from build123d import *

# Parameters (mm, degrees)
SKETCH1_W                 = 134.5
SKETCH1_H                 = 85
BOSS_EXTRUDE1_DEPTH       = 3
SKETCH2_W                 = 140.5
SKETCH2_H                 = 91
SKETCH2_W_2               = 134.5
SKETCH2_H_2               = 85
BOSS_EXTRUDE2_DEPTH       = 70
BOSS_EXTRUDE3_START       = 5
SKETCH3_W                 = 100
SKETCH3_H                 = 80
BOSS_EXTRUDE3_DEPTH       = 5
SKETCH5_W                 = 3
SKETCH5_H                 = 66
BOSS_EXTRUDE5_DEPTH       = 30
SKETCH6_R                 = 3
SKETCH6_R_2               = 1
BOSS_EXTRUDE6_DEPTH       = 10
SKETCH7_W                 = 100
SKETCH7_H                 = 80
CUT_EXTRUDE2_DEPTH        = 10
SKETCH6_2_R               = 3
SKETCH6_2_R_2             = 1
BOSS_EXTRUDE7_DEPTH       = 8
MIRROR4_COPY_1_SKETCH_R   = 3
MIRROR4_COPY_1_SKETCH_R_2 = 1
MIRROR4_COPY_1_DEPTH      = 8
SKETCH9_R                 = 26.15
SKETCH9_W                 = 29.3
SKETCH9_H                 = 26.2
SKETCH9_R_2               = 1
SKETCH9_R_3               = 3.4
SKETCH9_R_4               = 7.9
CUT_EXTRUDE3_DEPTH        = 3
SKETCH10_R                = 2.95
SKETCH10_R_2              = 5.9
CUT_EXTRUDE4_DEPTH        = 3
BOSS_EXTRUDE8_DEPTH       = 7
FILLET1_R                 = 4
CUT_EXTRUDE6_DEPTH        = 5


with BuildPart() as part:
    # Sketch1 → Boss-Extrude1 (new body)
    with BuildSketch(Plane(origin=(0, 0, 0), x_dir=(1, 0, 0), z_dir=(0, 1, 0))):
        with Locations((-12.25, 0)):
            Rectangle(SKETCH1_W, SKETCH1_H)
    extrude(amount=BOSS_EXTRUDE1_DEPTH)

    # Sketch2 → Boss-Extrude2 (add)
    with BuildSketch(Plane(origin=(0, 0, 0), x_dir=(1, 0, 0), z_dir=(0, 1, 0))):
        with Locations((-12.25, 0)):
            Rectangle(SKETCH2_W, SKETCH2_H)
        with Locations((-12.25, 0)):
            Rectangle(SKETCH2_W_2, SKETCH2_H_2, mode=Mode.SUBTRACT)
    extrude(amount=BOSS_EXTRUDE2_DEPTH)

    # Sketch5 → Boss-Extrude5 (add)
    with BuildSketch(Plane(origin=(0, 3, 0), x_dir=(1, 0, 0), z_dir=(0, 1, 0))):
        Polygon((-58, -26.5), (-58, -23.5), (-61, -23.5), (-79.5, -23.5), (-79.5, -26.5), align=None)
        with Locations((-59.5, 9.5)):
            Rectangle(SKETCH5_W, SKETCH5_H)
    extrude(amount=BOSS_EXTRUDE5_DEPTH)



with BuildPart() as body_2:
    # Sketch3 → Boss-Extrude3 (new body)
    with BuildSketch(Plane(origin=(0, 3, 0), x_dir=(1, 0, 0), z_dir=(0, 1, 0)).offset(BOSS_EXTRUDE3_START)):
        Rectangle(SKETCH3_W, SKETCH3_H)
    extrude(amount=BOSS_EXTRUDE3_DEPTH)


with BuildPart() as part_1:
    add(part.part)

    add(body_2.part)  # Boss-Extrude6 merges body 2
    # Sketch6 → Boss-Extrude6 (add)
    with BuildSketch(Plane(origin=(0, 3, 0), x_dir=(1, 0, 0), z_dir=(0, 1, 0))):
        with Locations((-45, -35)):
            Circle(SKETCH6_R)
        with Locations((-45, -35)):
            Circle(SKETCH6_R_2, mode=Mode.SUBTRACT)
    extrude(amount=BOSS_EXTRUDE6_DEPTH)

    # Sketch7 → Cut-Extrude2 (cut)
    with BuildSketch(Plane(origin=(0, 13, 0), x_dir=(1, 0, 0), z_dir=(0, 1, 0))):
        Rectangle(SKETCH7_W, SKETCH7_H)
    extrude(amount=-CUT_EXTRUDE2_DEPTH, mode=Mode.SUBTRACT)

    # Sketch6<2> → Boss-Extrude7 (add)
    with BuildSketch(Plane(origin=(0, 3, 0), x_dir=(1, 0, 0), z_dir=(0, 1, 0))):
        with Locations((-45, -35)):
            Circle(SKETCH6_2_R)
        with Locations((-45, -35)):
            Circle(SKETCH6_2_R_2, mode=Mode.SUBTRACT)
    boss_extrude7 = extrude(amount=BOSS_EXTRUDE7_DEPTH)

    # Mirror3: Boss-Extrude7 across plane
    add(boss_extrude7.mirror(Plane.XY))

    # Mirror4: Boss-Extrude7 across plane
    add(boss_extrude7.mirror(Plane(origin=(0, 0, 0), x_dir=(0, 0, 1), z_dir=(1, 0, 0))))

    # Mirror4 copy 1 sketch → Mirror4 copy 1 (add)
    with BuildSketch(Plane(origin=(0, 3, 0), x_dir=(-1, 0, 0), z_dir=(0, 1, 0))):
        with Locations((-45, -35)):
            Circle(MIRROR4_COPY_1_SKETCH_R)
        with Locations((-45, -35)):
            Circle(MIRROR4_COPY_1_SKETCH_R_2, mode=Mode.SUBTRACT)
    extrude(amount=MIRROR4_COPY_1_DEPTH)

    # Sketch9 → Cut-Extrude3 (cut)
    with BuildSketch(Plane.XY.offset(45.5)):
        with Locations((23, 40.85)):
            Circle(SKETCH9_R)
        with Locations((-47.5, 50)):
            Rectangle(SKETCH9_W, SKETCH9_H)
        with Locations((1.786796564, 62.063203436)):
            Circle(SKETCH9_R_2)
        with Locations((44.213203436, 62.063203436)):
            Circle(SKETCH9_R_2)
        with Locations((44.213203436, 19.636796564)):
            Circle(SKETCH9_R_2)
        with Locations((1.786796564, 19.636796564)):
            Circle(SKETCH9_R_2)
        with Locations((-58.75, 21.9)):
            Circle(SKETCH9_R_3)
        with Locations((-40.75, 21.9)):
            Circle(SKETCH9_R_4)
    extrude(amount=-CUT_EXTRUDE3_DEPTH, mode=Mode.SUBTRACT)

    # Sketch10 → Cut-Extrude4 (cut)
    with BuildSketch(Plane(origin=(58, 0, 0), x_dir=(0, 0, -1), z_dir=(1, 0, 0))):
        with Locations((15.5, 55)):
            Circle(SKETCH10_R)
        with Locations((30.5, 55)):
            Circle(SKETCH10_R_2)
    extrude(amount=-CUT_EXTRUDE4_DEPTH, mode=Mode.SUBTRACT)

    # Sketch11 → Boss-Extrude8 (add)
    with BuildSketch(Plane(origin=(0, 70, 0), x_dir=(1, 0, 0), z_dir=(0, 1, 0))):
        Polygon((-74.5, 42.5), (-79.5, 42.5), (-79.5, 37.5), align=None)
        Polygon((55, 37.5), (55, 42.5), (50, 42.5), align=None)
        Polygon((50, -42.5), (55, -42.5), (55, -37.5), align=None)
        Polygon((-79.5, -37.5), (-79.5, -42.5), (-74.5, -42.5), align=None)
    extrude(amount=-BOSS_EXTRUDE8_DEPTH)

    # Fillet1
    fillet1_edges = [part_1.edges().sort_by_distance(p)[0] for p in [
        (58, 35, 45.5),
        (58, 35, -45.5),
        (-82.5, 35, -45.5),
        (-82.5, 35, 45.5),
    ]]
    fillet(fillet1_edges, radius=FILLET1_R)

    # Sketch13 → Cut-Extrude6 (cut)
    with BuildSketch(Plane(origin=(0, 70, 0), x_dir=(1, 0, 0), z_dir=(0, 1, 0))):
        with BuildLine():
            ThreePointArc((55.371320344, 42.871320344), (53.957106781, 42.871320344), (53.957106781, 41.457106781))
            Line((53.957106781, 41.457106781), (55.371320344, 42.871320344))
        make_face()
        with BuildLine():
            Line((55.371320344, 42.871320344), (53.957106781, 41.457106781))
            ThreePointArc((53.957106781, 41.457106781), (55.046896995, 41.24033403), (55.664213562, 42.164213562))
            ThreePointArc((55.664213562, 42.164213562), (55.588093095, 42.546896995), (55.371320344, 42.871320344))
        make_face()
        with BuildLine():
            ThreePointArc((53.957106781, -41.457106781), (53.957106781, -42.871320344), (55.371320344, -42.871320344))
            Line((55.371320344, -42.871320344), (53.957106781, -41.457106781))
        make_face()
        with BuildLine():
            Line((53.957106781, -41.457106781), (55.371320344, -42.871320344))
            ThreePointArc((55.371320344, -42.871320344), (55.588093095, -42.546896995), (55.664213562, -42.164213562))
            ThreePointArc((55.664213562, -42.164213562), (55.046896995, -41.24033403), (53.957106781, -41.457106781))
        make_face()
        with BuildLine():
            ThreePointArc((-78.164213562, -42.164213562), (-78.24033403, -41.78153013), (-78.457106781, -41.457106781))
            Line((-78.457106781, -41.457106781), (-79.871320344, -42.871320344))
            ThreePointArc((-79.871320344, -42.871320344), (-78.78153013, -43.088093095), (-78.164213562, -42.164213562))
        make_face()
        with BuildLine():
            Line((-79.871320344, -42.871320344), (-78.457106781, -41.457106781))
            ThreePointArc((-78.457106781, -41.457106781), (-79.871320344, -41.457106781), (-79.871320344, -42.871320344))
        make_face()
        with BuildLine():
            ThreePointArc((-78.164213562, 42.164213562), (-78.78153013, 43.088093095), (-79.871320344, 42.871320344))
            Line((-79.871320344, 42.871320344), (-78.457106781, 41.457106781))
            ThreePointArc((-78.457106781, 41.457106781), (-78.24033403, 41.78153013), (-78.164213562, 42.164213562))
        make_face()
        with BuildLine():
            Line((-78.457106781, 41.457106781), (-79.871320344, 42.871320344))
            ThreePointArc((-79.871320344, 42.871320344), (-79.871320344, 41.457106781), (-78.457106781, 41.457106781))
        make_face()
    extrude(amount=-CUT_EXTRUDE6_DEPTH, mode=Mode.SUBTRACT)


solid = part_1.part
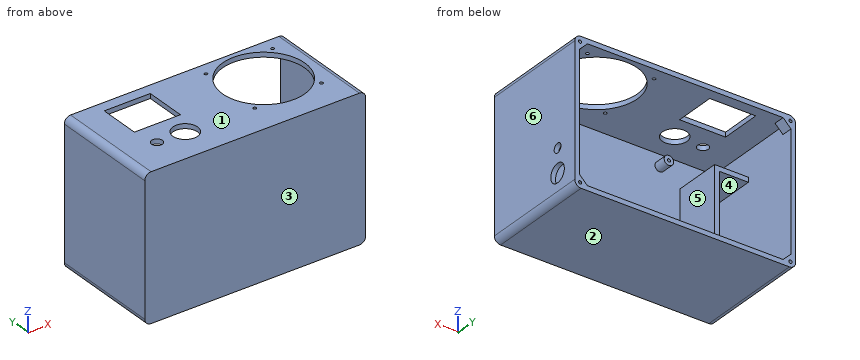
Could you check a few things on this model? Use its own coordinates, in mm. Face numbers are marked on the shaded views. A direction names the side the tool comes from. Give positions to 0.01 mm unless a question says otherwise; leave off trailing zeros. Loops run counter-clockwise (first coordinate to the right, second up) from the corner with the lowest first, then second, coordinate; pieces in that order, holes last. Notation, with made-up numbers: (-31, 63) -> (10, 63) arc R15 cw to (10, 84) -> close; hole circle Ø5 at (-29.75, -31). An arc over 180 degrees is marked (long way). Answer as CSV lines item,"result". Start each with the question number.
(1) If we section it at D-D on z = 9: Write out the boundary of the cut face in (x, y), then the cut area to 4 significant figures.
(2) We'd pull the mould along Z, two halves only. Please class the marked faces 1, 2, 3 and 4: released by +Z, released by -Z, zero draft, split by the parting line, or undercut.
(3) If we section it at C-C on x = 23: Write out the boundary of the cut face in (y, z), then the cut area to 3 significant figures.
(4) If we section it at A-A on y = 6: Count the separate pieces of the cut face and the enclosed holes in it, then the cut area to 3 significant figures.
(5) I need wall thicknesses on probe 1 along X at (y, z) = (6, 35); probe 2 along Z at (x, y) = (45, 7); probe 3 along X at (y, z) = (9, 3). Which ranges of each line are inside material? Lowest first, please.
(6) Which directions (+Z, -Z, +X, -X, +Y, -Y) give clear straight access to the entire face, cutting with the end or side of a thin tool? Please do the marked faces 5 and 6.
(7) I'm going to push flat-ended pins straight in: pin 1 Ø5 at (x, z) = (-46, 33.5) entering from +Y; pin 2 Ø15 at (x, z) = (-67.5, 4.5) entering from +Y; pin 3 Ø1.5 at (y, z) = (51, 44) entering from -X. Where does each tip first touch, or does it pass through?
(8) If we section it at B-B on z = -15.5: Write out the boundary of the cut face in (x, y).
Computed:
1,outline,"(-82.5, 0) -> (58, 0) -> (58, 70) -> (55, 70) -> (55, 3) -> (-58, 3) -> (-58, 33) -> (-61, 33) -> (-61, 3) -> (-79.5, 3) -> (-79.5, 70) -> (-82.5, 70) -> close"
1,area,"913.5 mm2"
2,face 1,"released by +Z"
2,face 2,"released by -Z"
2,face 3,"zero draft"
2,face 4,"undercut"
3,outline,"(0, -45.5) -> (70, -45.5) -> (70, -42.5) -> (3, -42.5) -> (3, 42.5) -> (14.7, 42.5) -> (14.7, 45.5) -> (0, 45.5) -> close; (67, 42.5) -> (70, 42.5) -> (70, 45.5) -> (67, 45.5) -> close"
3,area,"518 mm2"
4,separate pieces,"5"
4,enclosed holes,"6"
4,area,"1,700 mm2"
5,probe 1,"x = -82.5 to -79.5, -48 to -46, -44 to -42, 42 to 44, 46 to 48, 55 to 58"
5,probe 2,"z = -45.5 to -42.5, -38 to -36, -34 to -32, 32 to 34, 36 to 38, 42.5 to 45.5"
5,probe 3,"x = -82.5 to -79.5, -61 to -58, 55 to 58"
6,face 5,"+Y"
6,face 6,"+Z, -Z, +X, +Y, -Y"
7,pin 1,"stops at y = 11"
7,pin 2,"stops at y = 33"
7,pin 3,"stops at x = -82.1"
8,outline,"(-82.5, 0) -> (58, 0) -> (58, 52.05) -> (55, 52.05) -> (55, 3) -> (-58, 3) -> (-58, 33) -> (-61, 33) -> (-61, 3) -> (-79.5, 3) -> (-79.5, 70) -> (-82.5, 70) -> close; (55, 57.95) -> (58, 57.95) -> (58, 70) -> (55, 70) -> close"
